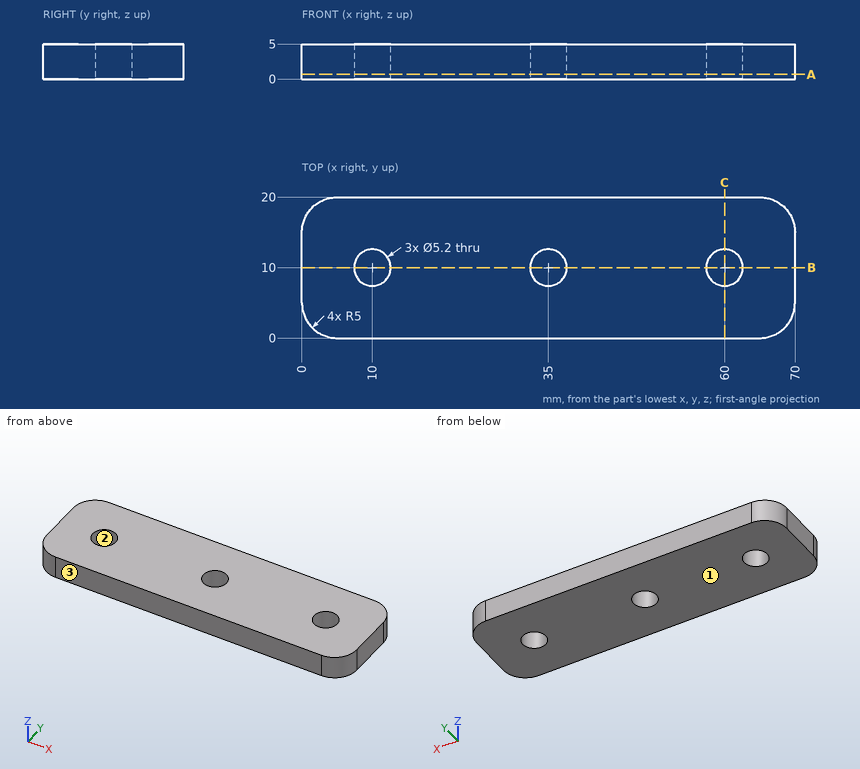
The figure shows three views and two pictorial views of one solid part (mm, origin at its lowest corner). Answer the questions. Coordinates: 2 decimals unless noted, no trailing zeros. Order: outer loops, then holes, each group sorted by start corner. A loop starts at its lowest first (then second) coordinate and runs counter-clockwise, first axis right, second up. Notation, with made-up numbers: (41.25, -3) - (96.25, -3) arc R18 ccw to (96.25, 30) - close; hole circle Ø4 at (7, -26). An arc over 180 degrees is marked (long way). Answer as a JSON object with one key per item and string values.
1. Each of these flat-tipped pins is pushed along its axis until it touches: P1, Ø10, axis at x = 62, y = 4.5, coming from the -Z side; P2, Ø4, axis at x = 10, y = 10, coming from the +Z side; P3, Ø3, axis at y = 3, z = 3.5, coming from the +X side. Where does it stop, or does it pass through?
Output values:
{"P1": "stops at z = 0", "P2": "passes through", "P3": "stops at x = 69.97"}
2. Find section C-C on x = 60. Determine the outline of the cut face in (y, z), plus the area to 3 significant figures.
Output values:
{"outline": "(0, 0) - (7.4, 0) - (7.4, 5) - (0, 5) - close; (12.6, 0) - (20, 0) - (20, 5) - (12.6, 5) - close", "area": "74.0 mm²"}
3. Consider line 1 (Y direction, x = 10, z = 3.1); line 2 (X direction, y = 11, z = 2.55); line 3 (X direction, y = 8.5, z = 1.35). Determine where each line is inside the solid, lowest interval first.
Output values:
{"line 1": "y = 0 to 7.4, 12.6 to 20", "line 2": "x = 0 to 7.6, 12.4 to 32.6, 37.4 to 57.6, 62.4 to 70", "line 3": "x = 0 to 7.88, 12.12 to 32.88, 37.12 to 57.88, 62.12 to 70"}
4. Find section B-B on y = 10. Determine the outline of the cut face in (x, z), plus the area to 3 significant figures.
Output values:
{"outline": "(0, 0) - (7.4, 0) - (7.4, 5) - (0, 5) - close; (12.6, 0) - (32.4, 0) - (32.4, 5) - (12.6, 5) - close; (37.6, 0) - (57.4, 0) - (57.4, 5) - (37.6, 5) - close; (62.6, 0) - (70, 0) - (70, 5) - (62.6, 5) - close", "area": "272 mm²"}
5. The mould has two halves that part along Y. Classify the marked faces 1, 2 and 3: +Y half, -Y half, draft (parallel to the pull), parting line (faces both ways), or undercut.
Output values:
{"face 1": "draft", "face 2": "undercut", "face 3": "-Y half"}
6. Find section A-A on z = 0.7. Determine the outline of the cut face in (x, y).
Output values:
{"outline": "(0, 5) arc R5 ccw to (5, 0) - (65, 0) arc R5 ccw to (70, 5) - (70, 15) arc R5 ccw to (65, 20) - (5, 20) arc R5 ccw to (0, 15) - close; hole circle Ø5.2 at (10, 10); hole circle Ø5.2 at (35, 10); hole circle Ø5.2 at (60, 10)"}
